Geometry: final body of the model. Coordinates: model frame, mm. Face numbers are marked on the shaded views. A direction names the side the tool comes from. Give positions to 0.01 mm unless a question says otherwise; leave off trailing zeros. Order: outer loops, then holes, each group sorted by start corner. A loop starts at its lowest first (then second) coordinate and runs counter-clockwise, first axis right, second up. Notation, with made-up numbers: (70, -12) - (76, -12) arc R29 ccw to (76, 26) - close; hole circle Ø5 at (2.25, 68). An arc over 180 degrees is marked (long way). Put each result on its own line as item: value. Start each with the question number.
1. Ray query, line 1 along Y through (x, z) = (-99.07, 7.85); line 2 along X through (y, z) = (-43.5, 1); line 3 along Y through (x, z) = (-71.5, 3). Return the intervals inside material, ascending. Write a range as from..to.
2. Section B-B on x = -75.5. Return the cut outline in (y, z), plus the area to 3 significant figures.
3. First-contact query: P1, Ø8, axis at x = -51.93, y = -75.9, coming from the -Z side. Flat tip, straight axial feed; report the tip coordinate or a pass-through.
4. Section C-C on y = -54.5. Return the cut outline in (x, z), plus the area to 3 significant figures.
5. Set-up query: the marked faces 1 and 2. Return all of +Z, -Z, +X, -X, +Y, -Y with unobstructed straight access to the full face (end or side cutting, diameter ignored); none if empty.
6. Section A-A on z = 5. Return the cut outline in (x, y), plus the area to 3 significant figures.
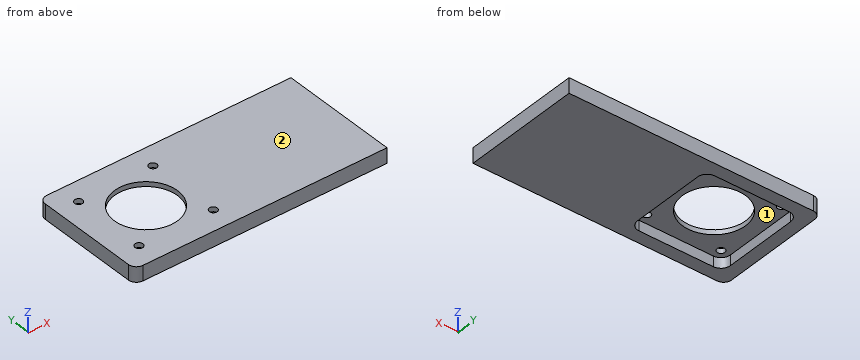
Autodesk Inventor part; units mm, degrees
ref_plane "YZ Plane" through (0, 0, 0) normal (1, 0, 0) x (0, 1, 0)
ref_plane "XZ Plane" through (0, 0, 0) normal (0, 1, 0) x (-1, 0, 0)
ref_plane "XY Plane" through (0, 0, 0) normal (0, 0, 1) x (1, 0, 0)
sketch "Esboço1" plane through (0, 0, 0) normal (0, 0, 1) x (1, 0, 0)
  line L0 (-33, -50) -> (-33, 950)
  line L1 (47, -50) -> (47, 950)
  line L2 (-113, -89.8276) -> (47, -89.8276)
  line L3 (47, -14.8276) -> (-113, -14.8276)
  line L4 (-113, -14.8276) -> (-113, -89.8276)
  line L5 (47, -89.8276) -> (47, -14.8276)
  point P0 (0, 0)
  dimension "d0" = 160
  dimension "d1" = 160
  dimension "d2" = 75
extrude "Extrusão1" add sketch "Esboço1" along normal blind 9.52
sketch "Esboço9" plane through (0, 0, 0) normal (0, 0, -1) x (-1, 0, 0)
  line L0 (105, -22.8276) -> (46, -22.8276)
  line L1 (46, -22.8276) -> (46, -81.8276)
  line L2 (46, -81.8276) -> (105, -81.8276)
  line L3 (105, -81.8276) -> (105, -22.8276)
  line L4 (105, -22.8276) -> (46, -81.8276) construction
  line L5 (46, -22.8276) -> (105, -81.8276) construction
  line L6 (105, -52.3276) -> (46, -52.3276) construction
  line L7 (75.5, -22.8276) -> (75.5, -81.8276) construction
  circle A0 centre (99.07, -28.7576) radius 2.5
  circle A1 centre (99.07, -75.8976) radius 2.5
  circle A2 centre (51.93, -28.7576) radius 2.5
  circle A3 centre (51.93, -75.8976) radius 2.5
  line L8 (113, -14.8276) -> (113, -89.8276)
  line L9 (113, -89.8276) -> (-47, -89.8276)
  circle A4 centre (75.5, -52.3276) radius 20
  point P0 (0, 0)
  dimension "d72" = 59
  dimension "d73" = 59
  dimension "d74" = 5
  dimension "d75" = 5
  dimension "d76" = 5
  dimension "d77" = 5
  dimension "d78" = 23.57
  dimension "d79" = 23.57
  dimension "d80" = 23.57
  dimension "d81" = 23.57
  dimension "d82" = 23.57
  dimension "d83" = 23.57
  dimension "d84" = 23.57
  dimension "d85" = 23.57
  dimension "d86" = 8
  dimension "d87" = 8
  dimension "d88" = 40
extrude "Extrusão6" cut sketch "Esboço9" against normal blind 6.52
sketch "Esboço10" plane through (-75.5, -52.3276, 0) normal (0, 0, -1) x (-1, 0, 0)
  circle A0 centre (0, 0) radius 20
  circle A1 centre (0, 0) radius 20
  circle A2 centre (23.57, -23.57) radius 2.5
  circle A3 centre (23.57, -23.57) radius 2.5
  circle A4 centre (23.57, 23.57) radius 2.5
  circle A5 centre (23.57, 23.57) radius 2.5
  circle A6 centre (-23.57, 23.57) radius 2.5
  circle A7 centre (-23.57, 23.57) radius 2.5
  circle A8 centre (-23.57, -23.57) radius 2.5
  circle A9 centre (-23.57, -23.57) radius 2.5
  point P0 (-75.5, 52.3276)
extrude "Extrusão7" cut sketch "Esboço10" against normal through all
fillet "Arredondamento1" radius 6 4 edges at (-105, -22.8276, 3.26) (-105, -81.8276, 3.26) (-46, -22.8276, 3.26) (-46, -81.8276, 3.26)
fillet "Arredondamento2" radius 5 2 edges at (-113, -14.8276, 4.76) (-113, -89.8276, 4.76)
equation "\"d0\" = d1"
equation "\"d79\" = d78"
equation "\"d80\" = d78"
equation "\"d81\" = d78"
equation "\"d82\" = d78"
equation "\"d83\" = d78"
equation "\"d84\" = d78"
equation "\"d85\" = d78"
properties part number "SUPORTE_MOTOR_EIXO_X"
Resolved:
1. line 1: -89.83..-78.4, -73.4..-31.26, -26.26..-14.83
1. line 2: -113..-105, -46..47
1. line 3: -89.83..-81.83, -22.83..-14.83
2. outline: (-89.83, 0) - (-81.83, 0) - (-81.83, 6.52) - (-72.33, 6.52) - (-72.33, 9.52) - (-89.83, 9.52) - close; (-32.33, 6.52) - (-22.83, 6.52) - (-22.83, 0) - (-14.83, 0) - (-14.83, 9.52) - (-32.33, 9.52) - close
2. area: 209 mm^2
3. P1: z = 6.52
4. outline: (-113, 0) - (-105, 0) - (-105, 6.52) - (-95.38, 6.52) - (-95.38, 9.52) - (-113, 9.52) - close; (-55.62, 6.52) - (-46, 6.52) - (-46, 0) - (47, 0) - (47, 9.52) - (-55.62, 9.52) - close
4. area: 1,020 mm^2
5. face 1: -Z
5. face 2: +Z, +X, -X, +Y, -Y
6. outline: (-113, -84.83) arc R5 ccw to (-108, -89.83) - (47, -89.83) - (47, -14.83) - (-108, -14.83) arc R5 ccw to (-113, -19.83) - close; hole (-105, -75.83) arc R6 ccw to (-99, -81.83) - (-52, -81.83) arc R6 ccw to (-46, -75.83) - (-46, -28.83) arc R6 ccw to (-52, -22.83) - (-99, -22.83) arc R6 ccw to (-105, -28.83) - close
6. area: 8,540 mm^2
